Read the model definition and answer for the solid it produces. Units are mm, in the model's axes. Round coordinates to 2 decimals unless told otherwise and drop trailing zeros. Loops run counter-clockwise (first coordinate to the right, second up) from the corner with the lowest first, then second, coordinate; pieces in that order, holes last. Notation, with made-up numbers: M 82.25,0.25 L 112.25,0.25 A18 cw 112.25,6.25 Z; hole C 60.25,75 d2. An arc over 180 degrees is marked long. Write each question's results on one line, items separated by ' | '.
from build123d import *

# Parameters (mm, degrees)
BOSS_EXTRUDE1_DEPTH                  = 19.05
F_3_8_CLEARANCE_HOLE1_D              = 10.31748
HOLE1_D                              = 3.175
HOLE1_DEPTH                          = 50.8
HOLE1_CSINK_D                        = 10.16
HOLE1_CSINK_ANGLE                    = 82
HOLE1_TIP                            = 0.953866233
F_15_64_0_23438_DIAMETER_HOLE1_D     = 5.953252
F_15_64_0_23438_DIAMETER_HOLE1_DEPTH = 23.611462659
F_15_64_0_23438_DIAMETER_HOLE1_TIP   = 1.788537341
FILLET1_R                            = 6.35


with BuildPart() as part:
    # Sketch1 → Boss-Extrude1 (new body)
    with BuildSketch(Plane.XY):
        Polygon((82.03946, -5024.878404071), (82.03946, -5533.415502988), (228.088766336, -5533.415502988), (228.088766336, -5447.34166837), (209.03946, -5142.552766987), (209.03946, -5024.878404071), align=None)
    extrude(amount=BOSS_EXTRUDE1_DEPTH)

    # 3/8 Clearance Hole1 (through all)
    with Locations(Plane.XY.offset(19.05)):
        with Locations((138.550999994, -5387.96381451), (138.550999994, -5164.31681451)):
            Hole(F_3_8_CLEARANCE_HOLE1_D / 2)

    # Hole1
    with Locations(Plane(origin=(0, -5562.870276207, 19.05), x_dir=(1, 0, 0), z_dir=(0, 0, 1))):
        with Locations((218.563766336, 102.817509219), (218.563766336, 48.504773219), (202.68946, 123.306744588), (202.68946, 317.949308361), (202.68946, 518.941872135), (88.38946, 518.941872135), (88.38946, 317.949308361), (88.38946, 123.306744588), (104.263766336, 216.849631358), (104.263766336, 132.677202288), (104.263766336, 48.504773219), (-104.263766336, 48.504773219), (-104.263766336, 132.677202288), (-104.263766336, 216.849631358), (-88.38946, 123.306744588), (-88.38946, 317.949308361), (-88.38946, 518.941872135), (-202.68946, 518.941872135), (-202.68946, 317.949308361), (-202.68946, 123.306744588), (-218.563766336, 48.504773219), (-218.563766336, 102.817509219)):
            CounterSinkHole(HOLE1_D / 2, HOLE1_CSINK_D / 2, depth=HOLE1_DEPTH, counter_sink_angle=HOLE1_CSINK_ANGLE)
            with Locations((0, 0, -(HOLE1_DEPTH + HOLE1_TIP / 2))):  # 118° drill point
                Cone(0, HOLE1_D / 2, HOLE1_TIP, mode=Mode.SUBTRACT)

    # 15/64 (0.23438) Diameter Hole1
    with Locations(Plane(origin=(209.03946, 0, 0), x_dir=(0, 0, -1), z_dir=(1, 0, 0))):
        with Locations((-9.526574029, -5089.226125561)):
            Hole(F_15_64_0_23438_DIAMETER_HOLE1_D / 2, depth=F_15_64_0_23438_DIAMETER_HOLE1_DEPTH)
            with Locations((0, 0, -(F_15_64_0_23438_DIAMETER_HOLE1_DEPTH + F_15_64_0_23438_DIAMETER_HOLE1_TIP / 2))):  # 118° drill point
                Cone(0, F_15_64_0_23438_DIAMETER_HOLE1_D / 2, F_15_64_0_23438_DIAMETER_HOLE1_TIP, mode=Mode.SUBTRACT)

    # Fillet1
    fillet1_edges = [part.edges().sort_by_distance(p)[0] for p in [
        (145.53946, -5024.878404071, 19.05),
    ]]
    fillet(fillet1_edges, radius=FILLET1_R)


solid = part.part
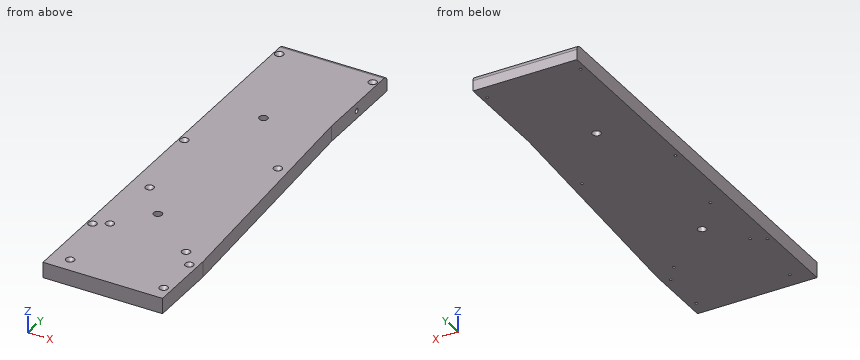
Item 1: The part is cut by section B-B (y = -5109.5). Determine the outline of the cut face in (x, z), plus the area to 3 significant figures.
Outcome:
outline: M 82.04,0 L 209.04,0 L 209.04,19.05 L 82.04,19.05 Z | area: 2,420 mm2
Item 2: The part is cut by section A-A (z = 3.25). State how many separate pieces and enclosed holes the cut face has, plus the area to 3 significant figures.
Outcome:
separate pieces: 1 | enclosed holes: 13 | area: 68,900 mm2
Item 3: Straight lines are drawn through the part: line 1 (Y direction, x = 89, z = 10.75); line 2 (Y direction, x = 125, z = 13); line 3 (X direction, y = -5388, z = 8.25). For each, find the intervals that lie inside material, in ascending order.
Outcome:
line 1: y = -5533.42 to -5441.03, -5438.1 to -5246.39, -5243.46 to -5045.39, -5042.46 to -5024.88 | line 2: y = -5533.42 to -5024.89 | line 3: x = 82.04 to 133.39, 143.71 to 224.38
Item 4: Flat-ended cylindrical pins translate along their axes: pin 1 (5 mm diameter, centred on x = 218.56, y = -5460.05, fed in from +Z); pin 2 (5 mm diameter, centred on x = 88.39, y = -5043.93, fed in from -Z); pin 3 (5 mm diameter, centred on y = -5353, z = 14, fed in from +X); pin 4 (3.5 mm diameter, centred on x = 202.69, y = -5043.93, fed in from +Z). Find the tip coordinate at first contact, or state that the pin passes through.
Outcome:
pin 1: stops at z = 16.09 | pin 2: stops at z = 0 | pin 3: stops at x = 222.35 | pin 4: stops at z = 15.22
Item 5: The part is cut by section C-C (y = -5269). Determine the outline of the cut face in (x, z).
Outcome:
outline: M 82.04,0 L 216.94,0 L 216.94,19.05 L 82.04,19.05 Z
